Source: CAD feature listing. Evaluate the final solid. Frame: model axes, mm. A direction names the side the tool comes from. Give positions to 0.01 mm unless a question says otherwise; leave off trailing zeros. Write each loop counter-clockwise with the first axis right and the second up, starting at its lowest first coordinate (ties: lowest second). Pieces come first, ordered by that corner, then holes. Notation, with made-up numbers: (0.5, 73) -> (58.5, 73) arc R16 ccw to (58.5, 91) -> close; hole circle Ø6 at (70, 4). An arc over 180 degrees is marked (long way). Write item = value, one per line.
from build123d import *

# Parameters (mm, degrees)
BOSS_EXTRU_1_DEPTH      = 4.5
ESQUISSE4_R             = 2.5
ENL_V_MAT_EXTRU_1_DEPTH = 0.1
ENL_V_START             = -0.1
ESQUISSE5_R             = 2.5
ENL_V_MAT_EXTRU_2_DEPTH = 0.1
ENL_V_MAT_EXTRU_3_DEPTH = 9.788771245
CONG_1_R                = 1
ESQUISSE7_W             = 1.6
ESQUISSE7_H             = 0.4
BOSS_EXTRU_4_DEPTH      = 1.5
ESQUISSE8_W             = 1
ESQUISSE8_H             = 0.4
BOSS_EXTRU_5_DEPTH      = 3.5
CHANFREIN3_SIZE         = 0.3
CHANFREIN4_SIZE         = 0.4


with BuildPart() as part:
    # Esquisse1 → Boss.-Extru.1 (new body)
    with BuildSketch(Plane.XY):
        with BuildLine():
            Line((-4, -3.243840317), (-4, -5.6))
            Line((-4, -5.6), (4, -5.6))
            Line((4, -5.6), (4, -3.243840317))
            ThreePointArc((4, -3.243840317), (0, 5.15), (-4, -3.243840317))
        make_face()
    extrude(amount=BOSS_EXTRU_1_DEPTH)

    # Esquisse4 → Enlèv. mat.-Extru.1 (cut)
    with BuildSketch(Plane(origin=(0, 0, 0), x_dir=(-1, 0, 0), z_dir=(0, 0, -1))):
        Circle(ESQUISSE4_R)
    extrude(amount=-ENL_V_MAT_EXTRU_1_DEPTH, mode=Mode.SUBTRACT)

    # Esquisse5 → Enlèv. mat.-Extru.2 (cut)
    with BuildSketch(Plane.XY.offset(4.5).offset(ENL_V_START)):
        with Locations(Location((0, 0, 0), (0, 0, 180))):
            Circle(ESQUISSE5_R)
    extrude(amount=ENL_V_MAT_EXTRU_2_DEPTH, mode=Mode.SUBTRACT)

    # Esquisse6 → Enlèv. mat.-Extru.3 (cut, through all)
    with BuildSketch(Plane(origin=(0, 0, 0.1), x_dir=(-1, 0, 0), z_dir=(0, 0, -1))):
        Polygon((0, 2), (-0.6, 1.4), (-0.3, 1.4), (-0.3, -2), (0.3, -2), (0.3, 1.4), (0.6, 1.4), align=None)
    extrude(amount=-ENL_V_MAT_EXTRU_3_DEPTH, mode=Mode.SUBTRACT)

    # Congé1
    cong_1_edges = [part.edges().sort_by_distance(p)[0] for p in [
        (4, -3.243840317, 2.25),
        (4, -5.6, 2.25),
        (-4, -5.6, 2.25),
        (-4, -3.243840317, 2.25),
    ]]
    fillet(cong_1_edges, radius=CONG_1_R)

    # Esquisse7 → Boss.-Extru.4 (add)
    with BuildSketch(Plane.XY.offset(4.5)):
        with Locations((-2.5, -5.2)):
            Rectangle(ESQUISSE7_W, ESQUISSE7_H)
        with Locations((2.5, -5.2)):
            Rectangle(ESQUISSE7_W, ESQUISSE7_H)
        with Locations((0, 4.8)):
            Rectangle(ESQUISSE7_W, ESQUISSE7_H)
    extrude(amount=BOSS_EXTRU_4_DEPTH)

    # Esquisse8 → Boss.-Extru.5 (add)
    with BuildSketch(Plane.XY.offset(6)):
        with Locations((0, 4.8)):
            Rectangle(ESQUISSE8_W, ESQUISSE8_H)
        with Locations((-2.5, -5.2)):
            Rectangle(ESQUISSE8_W, ESQUISSE8_H)
        with Locations((2.5, -5.2)):
            Rectangle(ESQUISSE8_W, ESQUISSE8_H)
    extrude(amount=BOSS_EXTRU_5_DEPTH)

    # Chanfrein3
    chanfrein3_edges = [part.edges().sort_by_distance(p)[0] for p in [
        (0.5, 4.8, 6),
        (-2, -5.2, 6),
        (3, -5.2, 6),
        (2, -5.2, 6),
        (-3, -5.2, 6),
        (-0.5, 4.8, 6),
    ]]
    chamfer(chanfrein3_edges, length=CHANFREIN3_SIZE - 0.0001)  # a hair under: the kernel refuses the full size

    # Chanfrein4
    chanfrein4_edges = [part.edges().sort_by_distance(p)[0] for p in [
        (-0.5, 4.8, 9.5),
        (0.5, 4.8, 9.5),
        (-3, -5.2, 9.5),
        (-2, -5.2, 9.5),
        (2, -5.2, 9.5),
        (3, -5.2, 9.5),
    ]]
    chamfer(chanfrein4_edges, length=CHANFREIN4_SIZE)


solid = part.part
1) Cut plane B-B (z = 5.75). Return the cut outline in (x, y).
Computed:
outline = (-3.3, -5.4) -> (-1.7, -5.4) -> (-1.7, -5) -> (-3.3, -5) -> close; (-0.8, 4.6) -> (0.8, 4.6) -> (0.8, 5) -> (-0.8, 5) -> close; (1.7, -5.4) -> (3.3, -5.4) -> (3.3, -5) -> (1.7, -5) -> close
2) Cut plane A-A (y = 0). Return the cut outline in (x, z).
Computed:
outline = (-5.15, 0) -> (-2.5, 0) -> (-2.5, 0.1) -> (-0.3, 0.1) -> (-0.3, 4.4) -> (-2.5, 4.4) -> (-2.5, 4.5) -> (-5.15, 4.5) -> close; (0.3, 0.1) -> (2.5, 0.1) -> (2.5, 0) -> (5.15, 0) -> (5.15, 4.5) -> (2.5, 4.5) -> (2.5, 4.4) -> (0.3, 4.4) -> close
3) Cut plane C-C (z = 2.75). Return the cut outline in (x, y), then the cut area to 3 significant figures.
Computed:
outline = (-4.19, -3) arc R1 cw to (-4, -3.58) -> (-4, -4.6) arc R1 ccw to (-3, -5.6) -> (3, -5.6) arc R1 ccw to (4, -4.6) -> (4, -3.58) arc R1 cw to (4.19, -3) arc R5.15 ccw (long way) to start; hole (-0.6, 1.4) -> (-0.3, 1.4) -> (-0.3, -2) -> (0.3, -2) -> (0.3, 1.4) -> (0.6, 1.4) -> (0, 2) -> close
area = 88.8 mm²
4) Access query for faces 1 (the flat face through (-4, -4, 2)), 2 (the flat face through (-1, 0, 4.4)), 3 (the flat face through (0, 4.6, 6)), 4 (the flat face through (0.3, 0, 2)), 5 (the flat face through (2, -5, 6)). Directions: +Z, -Z, +X, -X, +Y, -Y. A direction counts if a zero-diameter tool reaches every point of the face in a straight line with its end or side. Return the directions, or none.
Computed:
face_1 = +Z, -Z, -X, -Y
face_2 = +Z
face_3 = +Z, +X, -X, -Y
face_4 = +Z, -Z
face_5 = +Z, +X, -X, +Y
5) Material intervals for L1, parallel to Y at x = 0, z = 4.45; L2, parallel to Y at x = -1.25, z = 3.5; L3, parallel to Z at x = 2, y = -0.5, sorted ascending.
Computed:
L1 = -5.6 to -2.5, 2.5 to 5.15
L2 = -5.6 to 5
L3 = 0.1 to 4.4
6) Contact query for flat-ended pins moving along their axis: pin 1 (1.3 mm diameter, centred on x = -2.5, z = 8, fed in from +Y); pin 2 (6 mm diameter, centred on x = 3, y = -4, fed in from +Z); pin 3 (4 mm diameter, centred on x = 0, y = 0, fed in from +Z); pin 4 (4 mm diameter, centred on x = 0.5, z = 8, fed in from -Y). Output: stop coordinate, or through.
Computed:
pin_1 = -5
pin_2 = 9.5
pin_3 = 4.4
pin_4 = -5.4
7) Cut plane D-D (x = -1.5). Return the cut outline in (y, z), then the cut area to 3 significant figures.
Computed:
outline = (-5.6, 0) -> (-2, 0) -> (-2, 0.1) -> (2, 0.1) -> (2, 0) -> (4.93, 0) -> (4.93, 4.5) -> (2, 4.5) -> (2, 4.4) -> (-2, 4.4) -> (-2, 4.5) -> (-5.6, 4.5) -> close
area = 46.6 mm²
